Print and shaded views of the part. All mm, measured from the part's lowest x, y and z. A direction names the side the tool comes from. Round coordinates to 2 decimals unless told otherwise and drop trailing zeros. Order: outer loops, then holes, each group sorted by start corner. A loop starts at its lowest first (then second) coordinate and runs counter-clockwise, first axis right, second up. Notation, with made-up numbers: (2.25, -2.75) - (11.25, -2.75) arc R18 ccw to (11.25, 24.25) - close; hole circle Ø5 at (55.25, 38). An arc over 180 degrees is marked (long way). Write item = value, one per line.
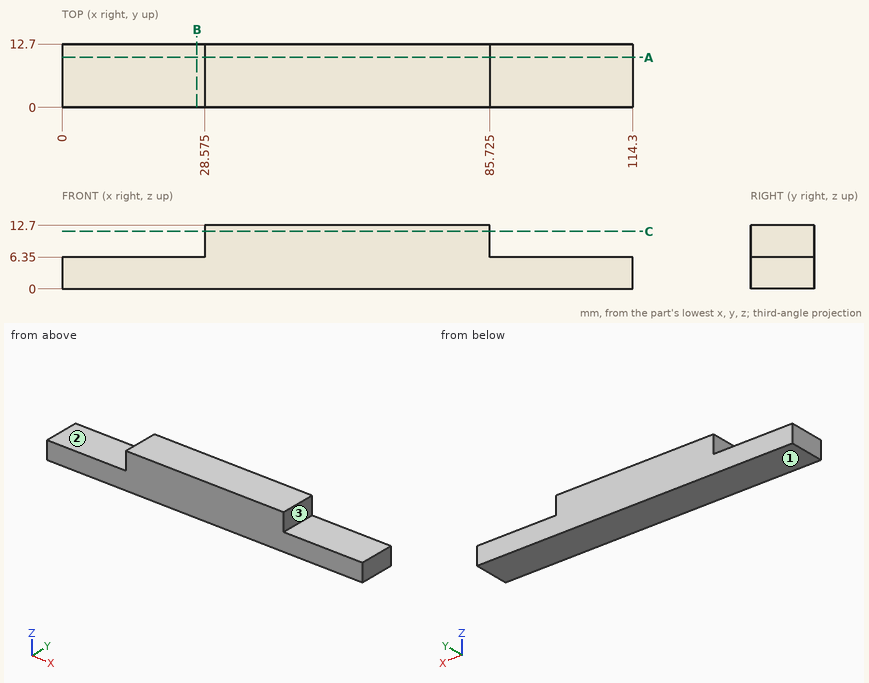
(1) Band-saw the part on B-B on x = 27. List the corners of the cut face in (y, z).
Solved:
outline = (0, 0) - (12.7, 0) - (12.7, 6.35) - (0, 6.35) - close
(2) Tool access for the marked faces 1, 2 and 3: list every direction of +Z, -Z, +X, -X, +Y, -Y with a clear straight run to the whole face (end or side of a thin tool).
Solved:
face_1 = -Z, +X, -X, +Y, -Y
face_2 = +Z, -X, +Y, -Y
face_3 = +Z, +X, +Y, -Y
(3) Band-saw the part on C-C on z = 11.5. List the corners of the cut face in (x, y) (3 decimals).
Solved:
outline = (28.575, 0) - (85.725, 0) - (85.725, 12.7) - (28.575, 12.7) - close
(4) Band-saw the part on A-A on y = 10. List the corners of the cut face in (x, z) (3 decimals).
Solved:
outline = (0, 0) - (114.3, 0) - (114.3, 6.35) - (85.725, 6.35) - (85.725, 12.7) - (28.575, 12.7) - (28.575, 6.35) - (0, 6.35) - close
(5) Probe line 1 along Z through (x, y) = (10, 6.75); line 2 along X through (y, z) = (1.75, 10.5) (3 decimals). List the from-to ranges inside material, lowest first.
Solved:
line_1 = 0 to 6.35
line_2 = 28.575 to 85.725
(6) Drop flat-ended pins along their axis: pin 1 (3 mm diameter, centred on y = 6.5, z = 9.5, fed in from -X) (3 decimals); pin 2 (4 mm diameter, centred on x = 107, y = 7.5, fed in from +Z). Give the stop position or say it passes through.
Solved:
pin_1 = 28.575
pin_2 = 6.35
